Design review of the part built by this model. Coordinates are the model's own, in mm. Face numbers are marked on the shaded views. A direction names the side the tool comes from. Coordinates: 2 decimals unless noted, no trailing zeros. Loops run counter-clockwise (first coordinate to the right, second up) from the corner with the lowest first, then second, coordinate; pieces in that order, holes last. Notation, with made-up numbers: (35.5, -38.75) -> (61.5, -38.75) arc R8 cw to (61.5, -34.75) -> close; hole circle Ø8 at (78.25, 68). An arc over 180 degrees is marked (long way). Use a Markdown table: item, result. Add a question column.
Q1. Clearance check with flat-ended pins moving along their axes: pin 1 Ø6 at (x, z) = (5, 12) entering from +Y; pin 2 Ø3 at (y, z) = (-3, 28.5) entering from +X; pin 3 Ø8 at (y, z) = (-11.5, 27.183) entering from +X; pin 4 Ø2 at (x, y) = (31.5, -3) entering from +Z. State where each tip first meets the part, or that it passes through.
Q2. Take a section at D-D on z = 26.5. Write out the cut boundary in (x, y).
Q3. For the marked faces 5, 6 and 7, list the 3-axis set-ups (+Z, -Z, +X, -X, +Y, -Y) from which the entire face can be reached by the end or side of a thin tool; tool diameter is ignored.
Q4. Take a section at B-B on y = -11.5. Write out the cut boundary in (x, z), plus the area to 3 significant figures.
Q5. Take a section at C-C on x = 28.5. Write out the cut boundary in (y, z).
Q6. Take a section at A-A on z = 8.7. Write out the cut boundary in (x, y).
Q7. Draft analysis for pull direction X (two halves, no side actions). For the marked faces 1, 2, 3 and 4, state which applies: pulls with the +X half, pulls with the -X half, needs draft (parallel to the pull), parting line crosses it, or undercut.
Q8. For probe 1 along Z at (x, y) = (19, -11.5); probe 2 along Z at (x, y) = (11.25, -11.5); probe 3 along X at (y, z) = (-6.5, 14), list the stretches that pass through material, from the lowest coordinate up.
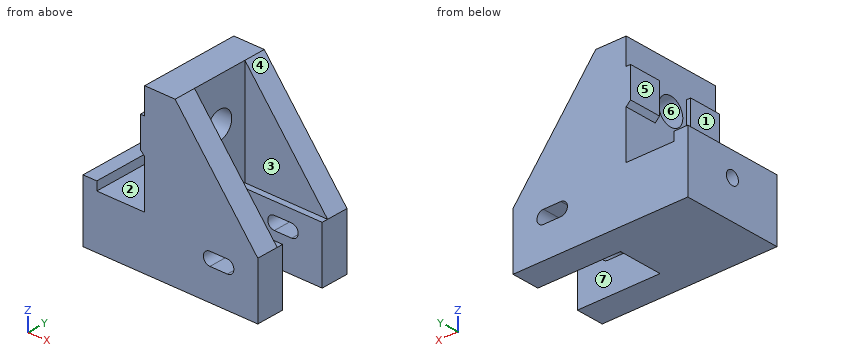
from build123d import *

# Parameters (mm, degrees)
F1_DEPTH = 23
F2_W     = 10.2
F2_H     = 13
F3_DEPTH = 19
F4_R     = 3.1
F5_DEPTH = 8
F7_DEPTH = 1
F8_R     = 1.55
F9_DEPTH = 21.162


with BuildPart() as f1:
    # F0 (on Front) → F1 (new body)
    with BuildSketch(Plane.XZ):
        Polygon((0, 14.2), (0, 0), (40.162, 0), (40.162, 13), (21.162, 37.2), (14.162, 37.2), (14.162, 31.2), (13.162, 31.2), (13.162, 24.2), (14.162, 23.2), (14.162, 12.2), (3.162, 12.2), (3.162, 14.2), align=None)
        with BuildLine():
            ThreePointArc((33.162, 10.2), (34.662, 8.7), (33.162, 7.2))
            Line((33.162, 7.2), (29.162, 7.2))
            ThreePointArc((29.162, 7.2), (27.662, 8.7), (29.162, 10.2))
            Line((29.162, 10.2), (33.162, 10.2))
        make_face(mode=Mode.SUBTRACT)
    extrude(amount=F1_DEPTH)

    # F2 (on face) → F3 (cut)
    with BuildSketch(Plane.YZ.offset(40.162)):
        Polygon((-18, 13), (-16.6, 13), (-6.4, 13), (-5, 13), (-5, 37.2), (-18, 37.2), align=None)
        with Locations((-11.5, 6.5)):
            Rectangle(F2_W, F2_H)
    extrude(amount=-F3_DEPTH, mode=Mode.SUBTRACT)

    # F4 (on face) → F5 (cut, through all)
    with BuildSketch(Plane.YZ.offset(21.162)):
        with Locations((-11.5, 27.183)):
            Circle(F4_R)
    extrude(amount=-F5_DEPTH, mode=Mode.SUBTRACT)

    # F6 (on face) → F7 (cut, through all)
    with BuildSketch(Plane(origin=(13.162, 0, 0), x_dir=(0, -1, 0), z_dir=(-1, 0, 0))):
        with BuildLine():
            Line((15.5000005274, 31.2), (7.5000005274, 31.2))
            Line((7.5000005274, 31.2), (7.5000005274, 24.2))
            Line((7.5000005274, 24.2), (10.6563703419, 24.2))
            ThreePointArc((10.6563703419, 24.2), (9.0276274613, 25.3128732583), (8.4, 27.183))
            ThreePointArc((8.4, 27.183), (13.3701267417, 29.6553725387), (12.3436296581, 24.2))
            Line((12.3436296581, 24.2), (15.5000005274, 24.2))
            Line((15.5000005274, 24.2), (15.5000005274, 31.2))
        make_face()
        with BuildLine():
            Line((10.6563703419, 24.2), (7.5000005274, 24.2))
            Line((7.5000005274, 24.2), (7.5000005274, 23.2))
            Line((7.5000005274, 23.2), (15.5000005274, 23.2))
            Line((15.5000005274, 23.2), (15.5000005274, 24.2))
            Line((15.5000005274, 24.2), (12.3436296581, 24.2))
            ThreePointArc((12.3436296581, 24.2), (13.3701267417, 29.6553725387), (8.4, 27.183))
            ThreePointArc((8.4, 27.183), (9.0276274613, 25.3128732583), (10.6563703419, 24.2))
        make_face()
    extrude(amount=-F7_DEPTH, mode=Mode.SUBTRACT)

    # F8 (on face) → F9 (cut, through all)
    with BuildSketch(Plane.YZ.offset(21.162)):
        with Locations((-11.5, 8.7000000016)):
            Circle(F8_R)
    extrude(amount=-F9_DEPTH, mode=Mode.SUBTRACT)


solid = f1.part
Answer list:
| question | item | result |
|---|---|---|
| 1 | pin 1 | y = 0 |
| 1 | pin 2 | x = 29.17 |
| 1 | pin 3 | x = 21.16 |
| 1 | pin 4 | z = 25.31 |
| 2 | outline | (13.16, -23) -> (29.56, -23) -> (29.56, -18) -> (21.16, -18) -> (21.16, -14.52) -> (14.16, -14.52) -> (14.16, -15.5) -> (13.16, -15.5) -> close; (13.16, -7.5) -> (14.16, -7.5) -> (14.16, -8.48) -> (21.16, -8.48) -> (21.16, -5) -> (29.56, -5) -> (29.56, 0) -> (13.16, 0) -> close |
| 3 | face 5 | +Z, -X, +Y, -Y |
| 3 | face 6 | +X, -X |
| 3 | face 7 | +Z, -Z, +X |
| 4 | outline | (0, 0) -> (21.16, 0) -> (21.16, 7.15) -> (0, 7.15) -> close; (0, 10.25) -> (21.16, 10.25) -> (21.16, 24.08) -> (14.16, 24.08) -> (14.16, 12.2) -> (3.16, 12.2) -> (3.16, 14.2) -> (0, 14.2) -> close; (14.16, 30.28) -> (21.16, 30.28) -> (21.16, 37.2) -> (14.16, 37.2) -> close |
| 4 | area | 330 mm² |
| 5 | outline | (-23, 0) -> (-16.6, 0) -> (-16.6, 7.35) -> (-23, 7.35) -> close; (-23, 10.05) -> (-16.6, 10.05) -> (-16.6, 13) -> (-18, 13) -> (-18, 27.85) -> (-23, 27.85) -> close; (-6.4, 0) -> (0, 0) -> (0, 7.35) -> (-6.4, 7.35) -> close; (-6.4, 10.05) -> (0, 10.05) -> (0, 27.85) -> (-5, 27.85) -> (-5, 13) -> (-6.4, 13) -> close |
| 6 | outline | (0, -23) -> (27.66, -23) -> (27.66, -16.6) -> (21.16, -16.6) -> (21.16, -13.05) -> (0, -13.05) -> close; (0, -9.95) -> (21.16, -9.95) -> (21.16, -6.4) -> (27.66, -6.4) -> (27.66, 0) -> (0, 0) -> close; (34.66, -23) -> (40.16, -23) -> (40.16, -16.6) -> (34.66, -16.6) -> close; (34.66, -6.4) -> (40.16, -6.4) -> (40.16, 0) -> (34.66, 0) -> close |
| 7 | face 1 | pulls with the -X half |
| 7 | face 2 | undercut |
| 7 | face 3 | needs draft |
| 7 | face 4 | pulls with the +X half |
| 8 | probe 1 | 0 to 7.15, 10.25 to 24.08, 30.28 to 37.2 |
| 8 | probe 2 | 0 to 7.15, 10.25 to 12.2 |
| 8 | probe 3 | 0 to 3.16, 14.16 to 21.16 |
